Autodesk Inventor part; units mm, degrees
ref_plane "Plan de construction1" through (0, 0, 1) normal (0, 0, -1) x (-1, 0, 0)
ref_plane "YZ Plane" through (0, 0, 0) normal (1, 0, 0) x (0, 1, 0)
ref_plane "XZ Plane" through (0, 0, 0) normal (0, 1, 0) x (-1, 0, 0)
sketch "Esquisse1" plane through (0, 0, 0) normal (0, 0, 1) x (1, 0, 0)
  circle A0 centre (0, 0) radius 17.5
  circle A1 centre (0, 0) radius 8.25
  dimension "d0" = 16.5
  dimension "d1" = 35
extrude "Extrusion1" add sketch "Esquisse1" along normal blind 8
chamfer "Chanfrein1" distance 0.5 angle 45 2 edges at (-8.25, 0, 0) (-8.25, 0, 8)
chamfer "Chanfrein2" distance 1 angle 45 2 edges at (-17.5, 0, 8) (-17.5, 0, 0)
ref_plane "Plan de construction1" through (0, 0, 1) normal (0, 0, -1) x (-1, 0, 0)
sketch "Esquisse3" plane through (0, 0, 1) normal (0, 0, -1) x (-1, 0, 0)
  circle A0 centre (0, 0) radius 17.5
  circle A1 centre (0, 0) radius 8.25
  line L0 (10.1036, 17.5) -> (20.2073, 0)
  line L1 (20.2073, 0) -> (10.1036, -17.5)
  line L2 (10.1036, -17.5) -> (-10.1036, -17.5)
  line L3 (-10.1036, -17.5) -> (-20.2073, 0)
  line L4 (-20.2073, 0) -> (-10.1036, 17.5)
  line L5 (-10.1036, 17.5) -> (10.1036, 17.5)
extrude "Extrusion2" add sketch "Esquisse3" against normal blind 6 contours A0 L0 L1 | A0 L5 L0 | L1 L2 A0 | A0 L4 L5 | L2 L3 A0 | A0 L3 L4
chamfer "Chanfrein3" distance 2 angle 45 6 edges at (10.1036, 17.5, 4) (20.2073, 0, 4) (10.1036, -17.5, 4) (-10.1036, -17.5, 4) (-20.2073, 0, 4) (-10.1036, 17.5, 4)
sketch "Esquisse4" plane through (-8.1036, -17.5, 1) normal (0, -1, 0) x (1, 0, 0)
  line L0 (16.2073, 6) -> (16.2073, 0)
  point P0 (8.1036, -1)
  point P1 (8.1036, 3)
  point P2 (16.2073, 3)
hole "Perçage1" at (0, -17.5, 4) direction (0, 1, 0) diameter 3.242 depth 6 tip angle 118
properties part number "support_canon_ext" material "Aluminium 6061"
Can you work these out from the model? Positions are in its coordinate system, mm. A direction names the side the tool comes from. Give positions to 0.01 mm unless a question says otherwise; leave off trailing zeros. Loops run counter-clockwise (first coordinate to the right, second up) from the corner with the lowest first, then second, coordinate; pieces in that order, holes last. Notation, with made-up numbers: (-37, -20) - (-26, -20) arc R18 cw to (-26, -7) - close; hole circle Ø11 at (17, 48.25). An arc over 180 degrees is marked (long way). Answer as a JSON object with one key per item and string values.
Q1. If I drill on L1, parallel to Y at x = -1.5, z = 2; L2, parallel to Y at x = 0, z = 3; L3, parallel to X at y = -3.5, z = 1.75, over which ranges is the centre line in solid material (lowest first)?
Geometry says:
{"L1": "-17.5 to -8.11, 8.11 to 17.5", "L2": "-11.13 to -8.25, 8.25 to 17.5", "L3": "-18.19 to -7.47, 7.47 to 18.19"}
Q2. Imagine slicing it at A-A on y = 0. Write out the boundary of the cut face in (x, z).
Geometry says:
{"outline": "(-19.21, 1) - (-17.5, 1) - (-16.5, 0) - (-8.75, 0) - (-8.25, 0.5) - (-8.25, 7.5) - (-8.75, 8) - (-16.5, 8) - (-17.5, 7) - (-19.21, 7) - close; (8.25, 0.5) - (8.75, 0) - (16.5, 0) - (17.5, 1) - (19.21, 1) - (19.21, 7) - (17.5, 7) - (16.5, 8) - (8.75, 8) - (8.25, 7.5) - close"}
Q3. If we mould it in two halves opening along Z, with no side actions, what happens to faces 3 (the flat face through (19.207, 0, 4)), 4 (the flat face through (-9.2, 15.4, 7)), 5 (the cylindrical face through (-0.07, -14.46, 5.62)), 6 (the flat face through (-9.2, -15.4, 1))? For each: pulls with the +Z half, pulls with the -Z half, needs draft (parallel to the pull), parting line crosses it, or undercut.
Geometry says:
{"face 3": "needs draft", "face 4": "pulls with the +Z half", "face 5": "undercut", "face 6": "pulls with the -Z half"}
Q4. Will these pins go through, and if not, where does the flat tip stop? P1, Ø3, axis at x = -13, z = 1, coming from the +Y side; P2, Ø1.2, axis at x = -17, y = -4.5, coming from the +Z side; P3, Ø1, axis at y = 3, z = 6.5, coming from the -X side.
Geometry says:
{"P1": "y = 15.08", "P2": "z = 7.51", "P3": "x = -18.76"}
Q5. Which directions (+Z, -Z, +X, -X, +Y, -Y) give clear straight access to the entire face, cutting with the end or side of a thin tool? Please do faces 1 (the flat face through (18, 0, 1)), 2 (the flat face through (-15.212, -8.652, 3.958)).
Geometry says:
{"face 1": "-Z, +X", "face 2": "+Z, -Z, -X, -Y"}
